Autodesk Fusion 360 part; units mm, degrees
sketch "Sketch1" plane through (0, 0, 0) normal (0, 0, 1) x (1, 0, 0)
  line L0 (17, 25) -> (-17, 25)
  line L1 (-17, 25) -> (-17, -25)
  line L2 (-17, -25) -> (17, -25)
  line L3 (17, -25) -> (17, 25)
  line L4 (17, 25) -> (-17, -25) construction
  line L5 (-17, 25) -> (17, -25) construction
  circle A0 centre (-13.5, 21.5) radius 1.45
  line L6 (-20, 0) -> (19, 0) construction
  circle A1 centre (-13.5, -21.5) radius 1.45
  line L7 (0, -29) -> (0, 26) construction
  circle A2 centre (13.5, -21.5) radius 1.45
  circle A3 centre (13.5, 16.4) radius 1.45
  line L8 (-4, 11) -> (11, 11)
  line L9 (11, 11) -> (11, -15)
  line L10 (11, -15) -> (-4, -15)
  line L11 (-4, -15) -> (-4, 11)
  dimension "d1" = 34
  dimension "d2" = 50
  dimension "d3" = 2.9
  dimension "d4" = 3.5
  dimension "d5" = 3.5
  dimension "d6" = 2.9
  dimension "d7" = 3.5
  dimension "d8" = 8.6
extrude "Extrude1" add sketch "Sketch1" along normal blind 1.6 contours L0 L1 L2 L3 | L8 L9 L10 L11
extrude "Extrude2" add sketch "Sketch1" along normal blind 5 contours L8 L9 L10 L11
sketch "Sketch2" plane through (0, 25, 0) normal (0, 1, 0) x (-1, 0, 0)
  line L0 (-17, 0) -> (17, 0)
  line L1 (17, 0) -> (17, 1.6)
  line L2 (17, 1.6) -> (-17, 1.6)
  line L3 (-17, 1.6) -> (-17, 0)
  line L4 (-6.1, -1.5) -> (-12.5, -1.5)
  line L5 (-12.5, -1.5) -> (-12.5, 4.9)
  line L6 (-12.5, 4.9) -> (-6.1, 4.9)
  line L7 (-6.1, 4.9) -> (-6.1, -1.5)
  line L8 (-17, 0) -> (17, 0)
  line L9 (-6.1, -1.5) -> (-12.5, 4.9) construction
  line L10 (-12.5, -1.5) -> (-6.1, 4.9) construction
  circle A0 centre (-9.3, 1.7) radius 3.1
  dimension "d13" = 6.4
  dimension "d14" = 6.4
  dimension "d15" = 4.5
  dimension "d16" = 1.5
  dimension "d17" = 6.2
extrude "Extrude3" add sketch "Sketch2" along normal blind 2 contours L0 L2 L5 L8 A0 | L0 L4 L5 L7 L8 A0 | L0 L2 L8 A0 | L0 L8 A0 | L2 L5 L6 L7 A0 | L0 L2 L7 L8 A0 | L2 A0
extrude "Extrude4" add sketch "Sketch2" along normal blind 10 contours L0 L2 L8 A0 | L0 L8 A0 | L2 A0
equation "d4 = 2 mm + 1.5 mm"
equation "d8 = 7.1 mm + 1.5 mm"
Verification items for the finished model (mm, model axes). A direction names the side the tool comes from. Round coordinates to 2 decimals unless told otherwise and drop trailing zeros. Loops run counter-clockwise (first coordinate to the right, second up) from the corner with the lowest first, then second, coordinate; pieces in that order, holes last. Notation, with made-up numbers: (64, 54.25) - (101, 54.25) arc R23 ccw to (101, 67.25) - close; hole circle Ø5 at (-23.5, -37.75). An arc over 180 degrees is marked (long way). Write item = value, one per line.
Q1. Sectioned sample at B-B on x = 13.5. Record the boundary of the cut face in (y, z), plus the area to 3 significant figures.
Here are the results:
outline = (-25, 0) - (-22.95, 0) - (-22.95, 1.6) - (-25, 1.6) - close; (-20.05, 0) - (14.95, 0) - (14.95, 1.6) - (-20.05, 1.6) - close; (17.85, 0) - (25, 0) - (25, 1.6) - (17.85, 1.6) - close
area = 70.7 mm^2
Q2. Material ranges on L1, parallel to Y at x = 13.5, z = 1; L2, parallel to Y at x = 14.5, z = 1.5; L3, parallel to Y at x = 8.5, z = 3.75, recorded low to high.
Here are the results:
L1 = -25 to -22.95, -20.05 to 14.95, 17.85 to 25
L2 = -25 to -22.55, -20.45 to 15.35, 17.45 to 25
L3 = -15 to 11, 25 to 35
Q3. Mould release check, pull along Y, two halves, no side actions. Record for faces 1 (the flat face through (0, 0, 0)), 2 (the cylindrical face through (13.186, -20.084, 0.789)), 3 (the flat face through (9, 35, 2)): +Y half, -Y half, draft (parallel to the pull), parting line (faces both ways), or undercut.
Here are the results:
face_1 = draft
face_2 = undercut
face_3 = +Y half
Q4. Tool access check on faces 4 (the flat face through (4, -15, 3)), 5 (the flat face through (9, 25, 3)), 6 (the flat face through (9, 26, 4.9)). Record the directions out of +Z, -Z, +X, -X, +Y, -Y that give a thin tool (end or side, any length) a straight path to the whole face; none if there is none.
Here are the results:
face_4 = +Z, +X, -X, -Y
face_5 = +Z, +X, -X
face_6 = +Z, +X, -X, +Y
Q5. Sectioned sample at A-A on y = 21.5. Record the boundary of the cut face in (x, z).
Here are the results:
outline = (-17, 0) - (-14.95, 0) - (-14.95, 1.6) - (-17, 1.6) - close; (-12.05, 0) - (17, 0) - (17, 1.6) - (-12.05, 1.6) - close
Q6. Sectioned sample at D-D on z = 2.75. Record the boundary of the cut face in (x, y), plus the area to 3 significant figures.
Here are the results:
outline = (-4, -15) - (11, -15) - (11, 11) - (-4, 11) - close; (6.1, 25) - (12.5, 25) - (12.5, 27) - (12.22, 27) - (12.22, 35) - (6.38, 35) - (6.38, 27) - (6.1, 27) - close
area = 449 mm^2
Q7. Sectioned sample at C-C on y = -21.5. Record the boundary of the cut face in (x, z), plus the area to 3 significant figures.
Here are the results:
outline = (-17, 0) - (-14.95, 0) - (-14.95, 1.6) - (-17, 1.6) - close; (-12.05, 0) - (12.05, 0) - (12.05, 1.6) - (-12.05, 1.6) - close; (14.95, 0) - (17, 0) - (17, 1.6) - (14.95, 1.6) - close
area = 45.1 mm^2
Q8. Depth check by flat-ended pin: pin 1 (3.5 mm diameter, centred on x = 9.5, z = 3.5, fed in from -Y); pin 2 (4.5 mm diameter, centred on x = -13.5, y = 21.5, fed in from -Z); pin 3 (1.6 mm diameter, centred on x = 9.5, z = -1, fed in from -Y). Enter the tip coordinate at first touch or a pass-through.
Here are the results:
pin_1 = -15
pin_2 = 0
pin_3 = 25
